```python
from build123d import *

# Parameters (mm, degrees)
CYLINDER_R     = 0.5
CYLINDER_DEPTH = 18
BOX_W          = 20
BOX_H          = 40
BOX_DEPTH      = 10


with BuildPart() as sphere007:
    # Sphere007 → Sphere007 (revolve)
    with BuildSketch(Plane(origin=(16, 25, 10), x_dir=(1, 0, 0), z_dir=(0, -1, 0))):
        with BuildLine():
            ThreePointArc((0, -2), (2, 0), (0, 2))
            Line((0, 2), (0, -2))
        make_face()
    revolve(axis=Axis((16, 25, 10), (0, 0, 1)))


with BuildPart() as sphere006:
    # Sphere006 → Sphere006 (revolve)
    with BuildSketch(Plane(origin=(4, 36, 10), x_dir=(1, 0, 0), z_dir=(0, -1, 0))):
        with BuildLine():
            ThreePointArc((0, -2), (2, 0), (0, 2))
            Line((0, 2), (0, -2))
        make_face()
    revolve(axis=Axis((4, 36, 10), (0, 0, 1)))


with BuildPart() as sphere005:
    # Sphere005 → Sphere005 (revolve)
    with BuildSketch(Plane(origin=(10, 31, 10), x_dir=(1, 0, 0), z_dir=(0, -1, 0))):
        with BuildLine():
            ThreePointArc((0, -2), (2, 0), (0, 2))
            Line((0, 2), (0, -2))
        make_face()
    revolve(axis=Axis((10, 31, 10), (0, 0, 1)))


with BuildPart() as fusion:
    # Fusion base: copy of Sphere005
    add(sphere005.part)

    # Fusion: union Sphere007, Sphere006
    add(sphere007.part)
    add(sphere006.part)


with BuildPart() as sphere002:
    # Sphere002 → Sphere002 (revolve)
    with BuildSketch(Plane(origin=(4, 16, 10), x_dir=(1, 0, 0), z_dir=(0, -1, 0))):
        with BuildLine():
            ThreePointArc((0, -2), (2, 0), (0, 2))
            Line((0, 2), (0, -2))
        make_face()
    revolve(axis=Axis((4, 16, 10), (0, 0, 1)))


with BuildPart() as sphere003:
    # Sphere003 → Sphere003 (revolve)
    with BuildSketch(Plane(origin=(16, 16, 10), x_dir=(1, 0, 0), z_dir=(0, -1, 0))):
        with BuildLine():
            ThreePointArc((0, -2), (2, 0), (0, 2))
            Line((0, 2), (0, -2))
        make_face()
    revolve(axis=Axis((16, 16, 10), (0, 0, 1)))


with BuildPart() as sphere004:
    # Sphere004 → Sphere004 (revolve)
    with BuildSketch(Plane(origin=(10, 10, 10), x_dir=(1, 0, 0), z_dir=(0, -1, 0))):
        with BuildLine():
            ThreePointArc((0, -2), (2, 0), (0, 2))
            Line((0, 2), (0, -2))
        make_face()
    revolve(axis=Axis((10, 10, 10), (0, 0, 1)))


with BuildPart() as sphere:
    # Sphere → Sphere (revolve)
    with BuildSketch(Plane(origin=(4, 4, 10), x_dir=(1, 0, 0), z_dir=(0, -1, 0))):
        with BuildLine():
            ThreePointArc((0, -2), (2, 0), (0, 2))
            Line((0, 2), (0, -2))
        make_face()
    revolve(axis=Axis((4, 4, 10), (0, 0, 1)))


with BuildPart() as sphere001:
    # Sphere001 → Sphere001 (revolve)
    with BuildSketch(Plane(origin=(16, 4, 10), x_dir=(1, 0, 0), z_dir=(0, -1, 0))):
        with BuildLine():
            ThreePointArc((0, -2), (2, 0), (0, 2))
            Line((0, 2), (0, -2))
        make_face()
    revolve(axis=Axis((16, 4, 10), (0, 0, 1)))


with BuildPart() as fusion001:
    # Fusion001 base: copy of Sphere005
    add(sphere005.part)

    # Fusion001: union Sphere007, Sphere006, Sphere002, Sphere003, Sphere004, Sphere, Sphere001
    add(sphere007.part)
    add(sphere006.part)
    add(sphere002.part)
    add(sphere003.part)
    add(sphere004.part)
    add(sphere.part)
    add(sphere001.part)


with BuildPart() as fusion002:
    # Cylinder → Cylinder (new body)
    with BuildSketch(Plane(origin=(1, 20.5, 10), x_dir=(0, 0, -1), z_dir=(1, 0, 0))):
        Circle(CYLINDER_R)
    extrude(amount=CYLINDER_DEPTH)

    # Fusion002: union Fusion, Fusion001
    add(fusion.part)
    add(fusion001.part)


with BuildPart() as obj1:
    # Box → Box (new body)
    with BuildSketch(Plane.XY):
        with Locations((10, 20)):
            Rectangle(BOX_W, BOX_H)
    extrude(amount=BOX_DEPTH)

    # Cut: cut Fusion002
    add(fusion002.part, mode=Mode.SUBTRACT)


solid = obj1.part
```
Work out the finished part from the listing and answer in its coordinate system (mm). Give positions to 0.01 mm unless a question says otherwise; leave off trailing zeros. Order: outer loops, then holes, each group sorted by start corner. A loop starts at its lowest first (then second) coordinate and runs counter-clockwise, first axis right, second up. Notation, with made-up numbers: (-37.75, 65.25) -> (1.25, 65.25) arc R29 cw to (1.25, 91.25) -> close; hole circle Ø2 at (45.5, 84.5). An arc over 180 degrees is marked (long way). Answer as CSV lines item,"result". Start each with the question number.
(1) Section A-A, the plane y = 20.5 is taken. Write down the section's boundary in (x, z).
(2) For a pull along X with two mould halves and no side action, classify faces 1 (the flat face through (10, 0, 5)), 2 (the flat face through (20, 20, 5)), 3 (the cylindrical face through (9.9, 20.5, 9.5)) as released by +X, released by -X, zero draft, split by the parting line, or undercut.
(3) Consider line 1 along Y through (x, z) = (15, 9); line 2 along Y through (x, z) = (3.25, 8.5); line 3 along X through (y, z) = (31.5, 8.5). Determine where each line is inside the solid, lowest interval first.
(4) Section B-B, the plane x = 15.5 is taken. Write down the section's boundary in (y, z), plus the area to 3 significant figures.
(5) Section C-C, the plane y = 3 is taken. Write down the section's boundary in (x, z), plus the area to 3 significant figures.
Entries:
1,outline,"(0, 0) -> (20, 0) -> (20, 10) -> (19, 10) -> (19, 9.5) -> (1, 9.5) -> (1, 10) -> (0, 10) -> close"
2,face 1,"zero draft"
2,face 2,"released by +X"
2,face 3,"undercut"
3,line 1,"0 to 2.59, 5.41 to 14.59, 17.41 to 23.59, 26.41 to 40"
3,line 2,"0 to 2.91, 5.09 to 14.91, 17.09 to 34.91, 37.09 to 40"
3,line 3,"0 to 8.78, 11.22 to 20"
4,outline,"(0, 0) -> (40, 0) -> (40, 10) -> (26.94, 10) arc R1.94 cw to (23.06, 10) -> (21, 10) arc R0.5 cw to (20, 10) -> (17.94, 10) arc R1.94 cw to (14.06, 10) -> (5.94, 10) arc R1.94 cw to (2.06, 10) -> (0, 10) -> close"
4,area,"382 mm²"
5,outline,"(0, 0) -> (20, 0) -> (20, 10) -> (17.73, 10) arc R1.73 cw to (14.27, 10) -> (5.73, 10) arc R1.73 cw to (2.27, 10) -> (0, 10) -> close"
5,area,"191 mm²"
